Geometry check sheet. Reference: the model listing, model coordinates, mm. Face numbers are marked on the shaded views. Coordinates: 2 decimals unless noted, no trailing zeros. Loops run counter-clockwise (first coordinate to the right, second up) from the corner with the lowest first, then second, coordinate; pieces in that order, holes last. Notation, with made-up numbers: (-13, 65.25) - (19, 65.25) arc R18 cw to (19, 94.25) - close; hole circle Ø3 at (18, 83). An arc over 180 degrees is marked (long way). Write each question's results on one line, items separated by ' | '. Start each with the question number.
(1) Sectioned sample at B-B (z = 11). Enter the section's corners in (x, y).
(2) Go/stop test with flat-tipped pins: pin 1 Ø8 at (x, z) = (51.5, 3) entering from -Y; pin 2 Ø4 at (y, z) = (21.5, -1.5) entering from -X; pin 3 Ø5 at (y, z) = (10.5, 14.5) entering from +X. Record where each tip stops, or that it passes through.
(3) Mould release check, pull along Y, two halves, no side actions. Record for the marked faces 1, 2 and 3: pulls with the +Y half, pulls with the -Y half, needs draft (parallel to the pull), parting line crosses it, or undercut.
(4) Sectioned sample at A-A (z = -4.5). Enter the section's corners in (x, y).
(5) Material ranges on probe 1 along Y at (x, z) = (0, -6); probe 2 along Z at (x, y) = (45.5, 16.5); probe 3 along Y at (x, z) = (60, -11.5), recorded low to high.
from build123d import *

# Parameters (mm, degrees)
F0_R     = 15
F0_R_2   = 7.5
F1_DEPTH = 20
F2_DEPTH = 20
F3_R     = 2
F4_SIZE  = 2


with BuildPart() as f1:
    # F0 (on Top) → F1 (new body)
    with BuildSketch(Plane.XY):
        with BuildLine():
            ThreePointArc((7.5, -29.047375), (23.717082, -18.371173), (30, 0))
            ThreePointArc((30, 0), (23.717082, 18.371173), (7.5, 29.047375))
            ThreePointArc((7.5, 29.047375), (-30, 0), (7.5, -29.047375))
        make_face()
        Circle(F0_R, mode=Mode.SUBTRACT)
        with BuildLine():
            ThreePointArc((7.5, 29.047375), (23.717082, 18.371173), (30, 0))
            ThreePointArc((30, 0), (23.717082, -18.371173), (7.5, -29.047375))
            Line((7.5, -29.047375), (63.75, -14.523688))
            ThreePointArc((63.75, -14.523688), (45, 0), (63.75, 14.523688))
            Line((63.75, 14.523688), (7.5, 29.047375))
        make_face()
        with BuildLine():
            ThreePointArc((75, 0), (71.858541, 9.185587), (63.75, 14.523688))
            ThreePointArc((63.75, 14.523688), (45, 0), (63.75, -14.523688))
            ThreePointArc((63.75, -14.523688), (71.858541, -9.185587), (75, 0))
        make_face()
        with Locations((60, 0)):
            Circle(F0_R_2, mode=Mode.SUBTRACT)
    extrude(amount=-F1_DEPTH)

    # F0 (on Top) → F2 (join)
    with BuildSketch(Plane.XY):
        with BuildLine():
            ThreePointArc((7.5, -29.047375), (23.717082, -18.371173), (30, 0))
            ThreePointArc((30, 0), (23.717082, 18.371173), (7.5, 29.047375))
            ThreePointArc((7.5, 29.047375), (-30, 0), (7.5, -29.047375))
        make_face()
        Circle(F0_R, mode=Mode.SUBTRACT)
    extrude(amount=F2_DEPTH)

    # F3
    f3_edges = [f1.edges().sort_by_distance(p)[0] for p in [
        (-7.5, 29.047375, 20),
        (-15, 0, 20),
        (-30, 0, -20),
        (35.625, -21.785531, -20),
        (75, 0, -20),
        (35.625, 21.785531, -20),
        (-15, 0, -20),
        (52.5, 0, -20),
    ]]
    fillet(f3_edges, radius=F3_R)

    # F4
    f4_edges = [f1.edges().sort_by_distance(p)[0] for p in [
        (52.5, 0, 0),
    ]]
    chamfer(f4_edges, length=F4_SIZE)


solid = f1.part
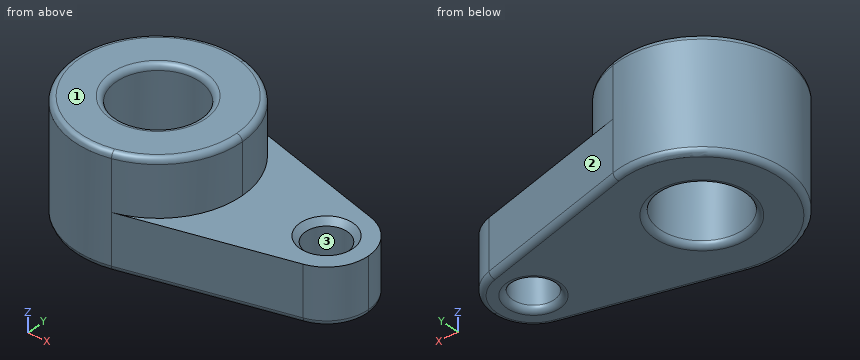
Outcome:
1) outline: (7.5, -29.05) arc R30 ccw to (30, 0) arc R30 ccw to (7.5, 29.05) arc R30 ccw (long way) to start; hole circle Ø30 at (0, 0)
2) pin 1: stops at y = -18.37 | pin 2: stops at x = -22.8 | pin 3: stops at x = 28.91
3) face 1: needs draft | face 2: pulls with the +Y half | face 3: undercut
4) outline: (7.5, -29.05) - (63.75, -14.52) arc R15 ccw to (63.75, 14.52) - (7.5, 29.05) arc R30 ccw (long way) to start; hole circle Ø30 at (0, 0); hole circle Ø15 at (60, 0)
5) probe 1: y = -30 to -15, 15 to 30 | probe 2: z = -20 to 0 | probe 3: y = -15.49 to -7.5, 7.5 to 15.49
